from build123d import *

# Parameters (mm, degrees)
SKETCH1_W                                           = 165
SKETCH1_H                                           = 90
BOSS_EXTRUDE1_DEPTH                                 = 7.5
CUT_EXTRUDE2_REACH                                  = 96.274
CBORE_START                                         = 1
CBORE_SLOT_FOR_M6_HEX_SOCKET_HEAD_CAP_SC_DEPTH      = 6.5
CBORE_SLOT_FOR_M6_HEX_SOCKET_HEAD_CA_3_DEPTH        = 1
FILLET1_R                                           = 5
CBORE_FOR_M6_HEX_SOCKET_HEAD_CAP_SCREW1_D           = 7
CBORE_FOR_M6_HEX_SOCKET_HEAD_CAP_SCREW1_CBORE_D     = 11
CBORE_FOR_M6_HEX_SOCKET_HEAD_CAP_SCREW1_CBORE_DEPTH = 6.5
CUT_EXTRUDE3_DEPTH                                  = 5
CUT_EXTRUDE4_REACH                                  = 96.274
SKETCH13_W                                          = 82.5
SKETCH13_H                                          = 90
CUT_EXTRUDE5_REACH                                  = 96.274
SKETCH14_W                                          = 0.5
SKETCH14_H                                          = 84.000354274


# Read off the part's stored shape, not the designer's step: CBORE SLOT for M6 Hex Socket Head Cap Screw1
with BuildPart() as part:
    # Sketch1 → Boss-Extrude1 (new body)
    with BuildSketch(Plane(origin=(0, 0, 0), x_dir=(1, 0, 0), z_dir=(0, 1, 0))):
        Rectangle(SKETCH1_W, SKETCH1_H)
    extrude(amount=BOSS_EXTRUDE1_DEPTH)

    # Sketch7 → Cut-Extrude2 (cut, up to next)
    with BuildSketch(Plane(origin=(0, 7.5, 0), x_dir=(1, 0, 0), z_dir=(0, 1, 0)), mode=Mode.PRIVATE) as cut_extrude2_sk1:
        with BuildLine():
            Line((-65, 45), (65, 45))
            ThreePointArc((65, 45), (0, 42), (-65, 45))
        make_face()
    cut_extrude2_tool1 = extrude(cut_extrude2_sk1.sketch, amount=-CUT_EXTRUDE2_REACH, mode=Mode.PRIVATE) & part.part
    # Sketch7 → Cut-Extrude2 (cut, up to next)
    with BuildSketch(Plane(origin=(0, 7.5, 0), x_dir=(1, 0, 0), z_dir=(0, 1, 0)), mode=Mode.PRIVATE) as cut_extrude2_sk2:
        with BuildLine():
            Line((-65, -45), (65, -45))
            ThreePointArc((65, -45), (0, -42), (-65, -45))
        make_face()
    cut_extrude2_tool2 = extrude(cut_extrude2_sk2.sketch, amount=-CUT_EXTRUDE2_REACH, mode=Mode.PRIVATE) & part.part
    add(cut_extrude2_tool1.solids().sort_by_distance((0, 7.5, -43.799781))[0], mode=Mode.SUBTRACT)
    add(cut_extrude2_tool2.solids().sort_by_distance((0, 7.5, 43.799781))[0], mode=Mode.SUBTRACT)

    # CBORE SLOT for M6 Hex Socket Head Ca 2 → CBORE SLOT for M6 Hex Socket Head Cap Screw1 (cut)
    with BuildSketch(Plane(origin=(0, 0, 0), x_dir=(1, 0, 0), z_dir=(0, 1, 0)).offset(CBORE_START)):
        with BuildLine():
            Line((80.5, -37.5), (80.5, -25))
            ThreePointArc((80.5, -25), (75, -19.5), (69.5, -25))
            Line((69.5, -25), (69.5, -37.5))
            ThreePointArc((69.5, -37.5), (75, -43), (80.5, -37.5))
        make_face()
        with BuildLine():
            ThreePointArc((80.5, 37.5), (75, 43), (69.5, 37.5))
            Line((69.5, 37.5), (69.5, 25))
            ThreePointArc((69.5, 25), (75, 19.5), (80.5, 25))
            Line((80.5, 25), (80.5, 37.5))
        make_face()
        with BuildLine():
            Line((-69.5, -37.5), (-69.5, -25))
            ThreePointArc((-69.5, -25), (-75, -19.5), (-80.5, -25))
            Line((-80.5, -25), (-80.5, -37.5))
            ThreePointArc((-80.5, -37.5), (-75, -43), (-69.5, -37.5))
        make_face()
        with BuildLine():
            ThreePointArc((-69.5, 37.5), (-75, 43), (-80.5, 37.5))
            Line((-80.5, 37.5), (-80.5, 25))
            ThreePointArc((-80.5, 25), (-75, 19.5), (-69.5, 25))
            Line((-69.5, 25), (-69.5, 37.5))
        make_face()
    extrude(amount=CBORE_SLOT_FOR_M6_HEX_SOCKET_HEAD_CAP_SC_DEPTH, mode=Mode.SUBTRACT)

    # CBORE SLOT for M6 Hex Socket Head Ca 3 o → CBORE SLOT for M6 Hex Socket Head Ca 3 (cut)
    with BuildSketch(Plane(origin=(0, 0, 0), x_dir=(1, 0, 0), z_dir=(0, 1, 0))):
        with BuildLine():
            Line((78.2, -37.5), (78.2, -25))
            ThreePointArc((78.2, -25), (75, -21.8), (71.8, -25))
            Line((71.8, -25), (71.8, -37.5))
            ThreePointArc((71.8, -37.5), (75, -40.7), (78.2, -37.5))
        make_face()
        with BuildLine():
            ThreePointArc((78.2, 37.5), (75, 40.7), (71.8, 37.5))
            Line((71.8, 37.5), (71.8, 25))
            ThreePointArc((71.8, 25), (75, 21.8), (78.2, 25))
            Line((78.2, 25), (78.2, 37.5))
        make_face()
        with BuildLine():
            Line((-71.8, -37.5), (-71.8, -25))
            ThreePointArc((-71.8, -25), (-75, -21.8), (-78.2, -25))
            Line((-78.2, -25), (-78.2, -37.5))
            ThreePointArc((-78.2, -37.5), (-75, -40.7), (-71.8, -37.5))
        make_face()
        with BuildLine():
            ThreePointArc((-71.8, 37.5), (-75, 40.7), (-78.2, 37.5))
            Line((-78.2, 37.5), (-78.2, 25))
            ThreePointArc((-78.2, 25), (-75, 21.8), (-71.8, 25))
            Line((-71.8, 25), (-71.8, 37.5))
        make_face()
    extrude(amount=CBORE_SLOT_FOR_M6_HEX_SOCKET_HEAD_CA_3_DEPTH, mode=Mode.SUBTRACT)

    # Fillet1
    fillet1_edges = [part.edges().sort_by_distance(p)[0] for p in [
        (82.5, 3.75, 45),
        (-82.5, 3.75, 45),
        (-82.5, 3.75, -45),
        (82.5, 3.75, -45),
    ]]
    fillet(fillet1_edges, radius=FILLET1_R)

    # CBORE for M6 Hex Socket Head Cap Screw1 (through all)
    with Locations(Plane.XZ):
        with Locations((-50, 0), (50, 0)):
            CounterBoreHole(CBORE_FOR_M6_HEX_SOCKET_HEAD_CAP_SCREW1_D / 2, CBORE_FOR_M6_HEX_SOCKET_HEAD_CAP_SCREW1_CBORE_D / 2, CBORE_FOR_M6_HEX_SOCKET_HEAD_CAP_SCREW1_CBORE_DEPTH)

    # Sketch12 → Cut-Extrude3 (cut)
    with BuildSketch(Plane(origin=(0, 7.5, 0), x_dir=(1, 0, 0), z_dir=(0, 1, 0))):
        with BuildLine():
            Line((-65, 45), (-65, 17.783744218))
            ThreePointArc((-65, 17.783744218), (-62.451932754, 10.782986997), (-56, 7.057961884))
            Line((-56, 7.057961884), (-44, 4.942038116))
            Line((-44, 4.942038116), (-44, -4.942038116))
            Line((-44, -4.942038116), (-56, -7.057961884))
            ThreePointArc((-56, -7.057961884), (-62.451932754, -10.782986997), (-65, -17.783744218))
            Line((-65, -17.783744218), (-65, -45))
            Line((-65, -45), (-20, -45))
            Line((-20, -45), (-20, 45))
            Line((-20, 45), (-65, 45))
        make_face()
        with BuildLine():
            Line((44, 4.942038116), (44, -4.942038116))
            Line((44, -4.942038116), (56, -7.057961884))
            ThreePointArc((56, -7.057961884), (62.451932754, -10.782986997), (65, -17.783744218))
            Line((65, -17.783744218), (65, -45))
            Line((65, -45), (20, -45))
            Line((20, -45), (20, 45))
            Line((20, 45), (65, 45))
            Line((65, 45), (65, 17.783744218))
            ThreePointArc((65, 17.783744218), (62.451932754, 10.782986997), (56, 7.057961884))
            Line((56, 7.057961884), (44, 4.942038116))
        make_face()
    extrude(amount=-CUT_EXTRUDE3_DEPTH, mode=Mode.SUBTRACT)

    # Sketch13 → Cut-Extrude4 (cut, up to next)
    with BuildSketch(Plane(origin=(0, 7.5, 0), x_dir=(1, 0, 0), z_dir=(0, 1, 0)), mode=Mode.PRIVATE) as cut_extrude4_sk1:
        with Locations((41.25, 0)):
            Rectangle(SKETCH13_W, SKETCH13_H)
    cut_extrude4_tool1 = extrude(cut_extrude4_sk1.sketch, amount=-CUT_EXTRUDE4_REACH, mode=Mode.PRIVATE) & part.part
    add(cut_extrude4_tool1.solids().sort_by_distance((41.25, 7.5, 0))[0], mode=Mode.SUBTRACT)

    # Sketch14 → Cut-Extrude5 (cut, up to next)
    with BuildSketch(Plane(origin=(0, 7.5, 0), x_dir=(1, 0, 0), z_dir=(0, 1, 0)), mode=Mode.PRIVATE) as cut_extrude5_sk1:
        with Locations((-0.25, 0)):
            Rectangle(SKETCH14_W, SKETCH14_H)
    cut_extrude5_tool1 = extrude(cut_extrude5_sk1.sketch, amount=-CUT_EXTRUDE5_REACH, mode=Mode.PRIVATE) & part.part
    add(cut_extrude5_tool1.solids().sort_by_distance((-0.25, 7.5, 0))[0], mode=Mode.SUBTRACT)


solid = part.part
Verification items for the finished model (mm, model axes). A direction names the side the tool comes from. Give positions to 0.01 mm unless a question says otherwise; leave off trailing zeros. Order: outer loops, then holes, each group sorted by start corner. A loop starts at its lowest first (then second) coordinate and runs counter-clockwise, first axis right, second up. Notation, with made-up numbers: M 79,-21.5 L 103,-21.5 A23 cw 103,2.5 Z; hole C -2,22 d4. An arc over 180 degrees is marked long. Answer as a JSON object with one key per item and string values. Group by question number.
1) Cross-section at C-C (x = -50). Enter the section's corners in (y, z), then the cut area to 3 significant figures.
2) Cross-section at B-B (y = 3.5). Enter the section's corners in (x, z), then the cut area to 3 significant figures.
3) Cross-section at A-A (z = 0). Enter the section's corners in (x, y), then the cut area to 4 significant figures.
4) Access from +Z, -Z, +X, -X, +Y, -Y to the whole of each face (thin tool, end or side, straight path). Record for faces 1 (the face through (-65, 5, 31)), 2 (the face through (-74.9, 0.5, -40.7)), 3 (the face through (-69.5, 4, -31)).
5) Cross-section at D-D (z = 13). Enter the section's corners in (x, y).
6) Mould release check, pull along X, two halves, no side actions. Record for faces 4 (the face through (-75, 4, 43)), 5 (the face through (-42, 0, -1)), 6 (the face through (-0.5, 4, 1)): released by +X, released by -X, zero draft, split by the parting line, or undercut.
7) Depth check by flat-ended pin: pin 1 Ø8 at (x, z) = (-38, 29.5) entering from +Y; pin 2 Ø3 at (x, y) = (-42, 4.5) entering from +Z; pin 3 Ø5.5 at (x, z) = (-52.5, -1) entering from -Y; pin 4 Ø8 at (x, z) = (-50, 0) entering from +Y. Enter the tip coordinate at first touch or a pass-through.
8) Scan lines: line 1 along X through (y, z) = (6.75, 30); line 2 along X through (y, z) = (6, 1); line 3 along Z through (x, y) = (-72, 2.5). Record each from-to range of solid material in increasing order. Write a range as [from, to].
Result sheet:
{
 "1": {"outline": "M 0,-43.77 L 2.5,-43.77 L 2.5,-6 L 7.5,-6 L 7.5,-3.5 L 6.5,-3.5 L 6.5,-5.5 L 0,-5.5 Z; M 0,5.5 L 6.5,5.5 L 6.5,3.5 L 7.5,3.5 L 7.5,6 L 2.5,6 L 2.5,43.77 L 0,43.77 Z", "area": "200 mm2"},
 "2": {"outline": "M -82.5,-40 A5 ccw -77.5,-45 L -65,-45 L -65,-17.78 A10.89 cw -56,-7.06 L -44,-4.94 L -44,4.94 L -56,7.06 A10.89 cw -65,17.78 L -65,45 L -77.5,45 A5 ccw -82.5,40 Z; M -20,-42.28 A705.67 cw -0.5,-42 L -0.5,42 A705.67 cw -20,42.28 Z; hole M -80.5,-37.5 A5.5 ccw -69.5,-37.5 L -69.5,-25 A5.5 ccw -80.5,-25 Z; hole M -80.5,25 A5.5 ccw -69.5,25 L -69.5,37.5 A5.5 ccw -80.5,37.5 Z; hole C -50,0 d11", "area": "2,960 mm2"},
 "3": {"outline": "M -82.5,0 L -55.5,0 L -55.5,6.5 L -53.5,6.5 L -53.5,7.5 L -82.5,7.5 Z; M -46.5,6.5 L -44.5,6.5 L -44.5,0 L -0.5,0 L -0.5,7.5 L -20,7.5 L -20,2.5 L -44,2.5 L -44,7.5 L -46.5,7.5 Z", "area": "416.5 mm2"},
 "4": {"face 1": "+Z, +Y", "face 2": "+Y, -Y", "face 3": "+Y"},
 "5": {"outline": "M -82.5,0 L -0.5,0 L -0.5,7.5 L -20,7.5 L -20,2.5 L -63.89,2.5 L -63.89,7.5 L -82.5,7.5 Z"},
 "6": {"face 4": "undercut", "face 5": "zero draft", "face 6": "released by +X"},
 "7": {"pin 1": "stops at y = 2.5", "pin 2": "passes through", "pin 3": "stops at y = 6.5", "pin 4": "stops at y = 7.5"},
 "8": {"line 1": "x = [-82.5, -80.5], [-69.5, -65], [-20, -0.5]", "line 2": "x = [-82.5, -55.41], [-44.59, -44], [-20, -0.5]", "line 3": "z = [-45, -42.11], [-20.39, 20.39], [42.11, 45]"}
}
